from build123d import *

# Parameters (mm, degrees)
SKETCH1_R           = 1.054
BOSS_EXTRUDE1_DEPTH = 3
SKETCH2_R           = 1.702
SKETCH2_R_2         = 0.65
CUT_EXTRUDE1_DEPTH  = 23.736281859


with BuildPart() as part:
    # Sketch1 → Boss-Extrude1 (new body)
    with BuildSketch(Plane(origin=(0, 0, 0), x_dir=(1, 0, 0), z_dir=(0, 1, 0))):
        with BuildLine():
            Line((0, 0), (9.035898385, 0))
            ThreePointArc((9.035898385, 0), (10.767949192, 1), (10.767949192, 3))
            Line((10.767949192, 3), (1.732050808, 18.650635095))
            ThreePointArc((1.732050808, 18.650635095), (0, 19.650635095), (-1.732050808, 18.650635095))
            Line((-1.732050808, 18.650635095), (-10.767949192, 3))
            ThreePointArc((-10.767949192, 3), (-10.767949192, 1), (-9.035898385, 0))
            Line((-9.035898385, 0), (0, 0))
        make_face()
        with Locations(Location((0, 17.650635095, 0), (0, 0, 270))):
            Circle(SKETCH1_R, mode=Mode.SUBTRACT)
        with Locations(Location((-9.035898385, 2, 0), (0, 0, 270))):
            Circle(SKETCH1_R, mode=Mode.SUBTRACT)
        with Locations(Location((9.035898385, 2, 0), (0, 0, 270))):
            Circle(SKETCH1_R, mode=Mode.SUBTRACT)
    extrude(amount=BOSS_EXTRUDE1_DEPTH)

    # Sketch2 → Cut-Extrude1 (cut, through all)
    with BuildSketch(Plane(origin=(0, 3, 0), x_dir=(1, 0, 0), z_dir=(0, 1, 0))):
        with Locations(Location((0, 10, 0), (0, 0, 270))):
            Circle(SKETCH2_R)
        with Locations(Location((0, 5, 0), (0, 0, 270))):
            Circle(SKETCH2_R_2)
    extrude(amount=-CUT_EXTRUDE1_DEPTH, mode=Mode.SUBTRACT)


solid = part.part
Design review of the part built by this model. Coordinates are the model's own, in mm. Give positions to 0.01 mm unless a question says otherwise; leave off trailing zeros. Loops run counter-clockwise (first coordinate to the right, second up) from the corner with the lowest first, then second, coordinate; pieces in that order, holes last. Notation, with made-up numbers: (-37.5, 9.5) - (7.5, 9.5) arc R25 ccw to (7.5, 29.5) - close; hole circle Ø8 at (17, 15). An arc over 180 degrees is marked (long way). Use CSV: the item, a comma, the result in double quotes. Start each with the question number.
1. Add section B-B (z = -2). State the section outline as (x, y) points, plus the area to 3 significant figures.
2. Add section D-D (z = -5). State the section outline as (x, y) points, plus the area to 3 significant figures.
3. Add section A-A (x = 0). State the section outline as (y, z) points.
4. Add section C-C (y = 0.25). State the section outline as (x, z) points, plus the area to 3 significant figures.
5. Draft analysis for pull direction Z (two halves, no side actions). For faces 1 (the flat face through (0, 3, -8)), 2 (the cylindrical face through (10.75, 1.48, -0.97)), 3 (the cylindrical face through (-0.404, 1.479, -16.677)), 4 (the cylindrical face through (0.03, 1.48, -19.65)), state which applies: released by +Z, released by -Z, zero draft, split by the parting line, or undercut.
6. Wall thickness on L1, parallel to X at y = 1, z = -2; L2, parallel to X at y = 2.85, z = -2.75; L3, parallel to Z at x = -9.75, y = 2.6: over which ranges is each line inside the solid? List them lowest first.
7. Insertion check: P1, Ø1.5, axis at y = 1, z = -4, coming from the -X side. The pin has a flat end and moves straight along its axis. Give the tip position at first contact, or say it passes through.
Results found:
1,outline,"(-11.04, 0) - (-10.09, 0) - (-10.09, 3) - (-11.04, 3) - close; (-7.98, 0) - (7.98, 0) - (7.98, 3) - (-7.98, 3) - close; (10.09, 0) - (11.04, 0) - (11.04, 3) - (10.09, 3) - close"
1,area,"53.6 mm²"
2,outline,"(-9.61, 0) - (-0.65, 0) - (-0.65, 3) - (-9.61, 3) - close; (0.65, 0) - (9.61, 0) - (9.61, 3) - (0.65, 3) - close"
2,area,"53.8 mm²"
3,outline,"(0, -19.65) - (3, -19.65) - (3, -18.7) - (0, -18.7) - close; (0, -16.6) - (3, -16.6) - (3, -11.7) - (0, -11.7) - close; (0, -8.3) - (3, -8.3) - (3, -5.65) - (0, -5.65) - close; (0, -4.35) - (3, -4.35) - (3, 0) - (0, 0) - close"
4,outline,"(-10.77, -3) - (-1.73, -18.65) arc R2 ccw to (1.73, -18.65) - (10.77, -3) arc R2 ccw to (9.04, 0) - (-9.04, 0) arc R2 ccw to start; hole circle Ø2.11 at (-9.04, -2); hole circle Ø3.4 at (0, -10); hole circle Ø2.11 at (0, -17.65); hole circle Ø1.3 at (0, -5); hole circle Ø2.11 at (9.04, -2)"
4,area,"242 mm²"
5,face 1,"zero draft"
5,face 2,"split by the parting line"
5,face 3,"undercut"
5,face 4,"released by -Z"
6,L1,"x = -11.04 to -10.09, -7.98 to 7.98, 10.09 to 11.04"
6,L2,"x = -10.89 to -9.78, -8.3 to 8.3, 9.78 to 10.89"
6,L3,"z = -4.76 to -2.78, -1.22 to -0.13"
7,P1,"stops at x = -10.62"
